```python
from build123d import *

# Parameters (mm, degrees)
F0_W     = 5
F0_H     = 5
F1_DEPTH = 3
F5_DEPTH = 5
F7_DEPTH = 7
F8_R     = 3.25
F9_DEPTH = 2


with BuildPart() as f1:
    # F0 (on Top) → F1 (new body)
    with BuildSketch(Plane.XY):
        with BuildLine():
            Line((2.5, 2.5), (5.4543560573, 2.5))
            ThreePointArc((5.4543560573, 2.5), (4.2426406871, 4.2426406871), (2.5, 5.4543560573))
            Line((2.5, 5.4543560573), (2.5, 2.5))
        make_face()
        with BuildLine():
            Line((2.5, -7.5), (2.5, -5.4543560573))
            ThreePointArc((2.5, -5.4543560573), (0, -6), (-2.5, -5.4543560573))
            Line((-2.5, -5.4543560573), (-2.5, -7.5))
            Line((-2.5, -7.5), (2.5, -7.5))
        make_face()
        with BuildLine():
            ThreePointArc((-5.4543560573, -2.5), (-4.2426406871, -4.2426406871), (-2.5, -5.4543560573))
            Line((-2.5, -5.4543560573), (-2.5, -2.5))
            Line((-2.5, -2.5), (-5.4543560573, -2.5))
        make_face()
        with BuildLine():
            ThreePointArc((-5.4543560573, -2.5), (-6, 0), (-5.4543560573, 2.5))
            Line((-5.4543560573, 2.5), (-7.5, 2.5))
            Line((-7.5, 2.5), (-7.5, -2.5))
            Line((-7.5, -2.5), (-5.4543560573, -2.5))
        make_face()
        with BuildLine():
            ThreePointArc((2.5, -5.4543560573), (4.2426406871, -4.2426406871), (5.4543560573, -2.5))
            Line((5.4543560573, -2.5), (2.5, -2.5))
            Line((2.5, -2.5), (2.5, -5.4543560573))
        make_face()
        with BuildLine():
            Line((-2.5, 2.5), (-2.5, 5.4543560573))
            ThreePointArc((-2.5, 5.4543560573), (-4.2426406871, 4.2426406871), (-5.4543560573, 2.5))
            Line((-5.4543560573, 2.5), (-2.5, 2.5))
        make_face()
        with BuildLine():
            ThreePointArc((5.4543560573, -2.5), (5.8620020617, -1.2794263668), (6, 0))
            ThreePointArc((6, 0), (5.8620020617, 1.2794263668), (5.4543560573, 2.5))
            Line((5.4543560573, 2.5), (2.5, 2.5))
            Line((2.5, 2.5), (2.5, -2.5))
            Line((2.5, -2.5), (5.4543560573, -2.5))
        make_face()
        Rectangle(F0_W, F0_H)
        with BuildLine():
            Line((-2.5, -2.5), (-2.5, 2.5))
            Line((-2.5, 2.5), (-5.4543560573, 2.5))
            ThreePointArc((-5.4543560573, 2.5), (-6, 0), (-5.4543560573, -2.5))
            Line((-5.4543560573, -2.5), (-2.5, -2.5))
        make_face()
        with BuildLine():
            Line((2.5, 2.5), (2.5, 5.4543560573))
            ThreePointArc((2.5, 5.4543560573), (0, 6), (-2.5, 5.4543560573))
            Line((-2.5, 5.4543560573), (-2.5, 2.5))
            Line((-2.5, 2.5), (2.5, 2.5))
        make_face()
        with BuildLine():
            ThreePointArc((-2.5, 5.4543560573), (0, 6), (2.5, 5.4543560573))
            Line((2.5, 5.4543560573), (2.5, 7.5))
            Line((2.5, 7.5), (-2.5, 7.5))
            Line((-2.5, 7.5), (-2.5, 5.4543560573))
        make_face()
        with BuildLine():
            ThreePointArc((5.4543560573, 2.5), (5.8620020617, 1.2794263668), (6, 0))
            ThreePointArc((6, 0), (5.8620020617, -1.2794263668), (5.4543560573, -2.5))
            Line((5.4543560573, -2.5), (7.5, -2.5))
            Line((7.5, -2.5), (7.5, 2.5))
            Line((7.5, 2.5), (5.4543560573, 2.5))
        make_face()
        with BuildLine():
            ThreePointArc((-2.5, -5.4543560573), (0, -6), (2.5, -5.4543560573))
            Line((2.5, -5.4543560573), (2.5, -2.5))
            Line((2.5, -2.5), (-2.5, -2.5))
            Line((-2.5, -2.5), (-2.5, -5.4543560573))
        make_face()
    extrude(amount=F1_DEPTH)

    # F5 (add): a face of the model
    f5_faces = [f1.faces().sort_by_distance(p)[0] for p in [
        (0, 0, 0),
    ]]
    extrude(f5_faces, amount=F5_DEPTH)


with BuildPart() as f4:
    # F3 (on Right) → F4 (revolve)
    with BuildSketch(Plane.YZ):
        with BuildLine():
            Line((0, -12), (0, 0))
            ThreePointArc((0, 0), (-6, -6), (0, -12))
        make_face()
    revolve(axis=Axis((0, 0, -6), (0, 0, -1)))


with BuildPart() as f1_1:
    add(f1.part)

    # F6: cut F4
    add(f4.part, mode=Mode.SUBTRACT)

    # F2 (on face) → F7 (join)
    with BuildSketch(Plane.XY.offset(3)):
        with BuildLine():
            ThreePointArc((-2.5, 5.4543560573), (-4.2426406871, 4.2426406871), (-5.4543560573, 2.5))
            Line((-5.4543560573, 2.5), (-7.5, 2.5))
            Line((-7.5, 2.5), (-7.5, -2.5))
            Line((-7.5, -2.5), (-5.4543560573, -2.5))
            ThreePointArc((-5.4543560573, -2.5), (-4.2426406871, -4.2426406871), (-2.5, -5.4543560573))
            Line((-2.5, -5.4543560573), (-2.5, -7.5))
            Line((-2.5, -7.5), (2.5, -7.5))
            Line((2.5, -7.5), (2.5, -5.4543560573))
            ThreePointArc((2.5, -5.4543560573), (4.2426406871, -4.2426406871), (5.4543560573, -2.5))
            Line((5.4543560573, -2.5), (7.5, -2.5))
            Line((7.5, -2.5), (7.5, 2.5))
            Line((7.5, 2.5), (5.4543560573, 2.5))
            ThreePointArc((5.4543560573, 2.5), (4.2426406871, 4.2426406871), (2.5, 5.4543560573))
            Line((2.5, 5.4543560573), (2.5, 7.5))
            Line((2.5, 7.5), (-2.5, 7.5))
            Line((-2.5, 7.5), (-2.5, 5.4543560573))
        make_face()
    extrude(amount=F7_DEPTH)

    # F8 (on face) → F9 (cut)
    with BuildSketch(Plane.XY.offset(10)):
        Circle(F8_R)
    extrude(amount=-F9_DEPTH, mode=Mode.SUBTRACT)


solid = f1_1.part
```
Geometry check sheet. Reference: the model listing, model coordinates, mm. A direction names the side the tool comes from. Round coordinates to 2 decimals unless told otherwise and drop trailing zeros. Loops run counter-clockwise (first coordinate to the right, second up) from the corner with the lowest first, then second, coordinate; pieces in that order, holes last. Notation, with made-up numbers: (-35.5, 25) - (-28.5, 25) arc R17 cw to (-28.5, 39) - close; hole circle Ø5 at (38, 14). An arc over 180 degrees is marked (long way). Write each question's results on one line, items separated by ' | '. Start each with the question number.
Q1. Cross-section at A-A on x = 0. Enter the section's corners in (y, z), and give its area (3 significant figures).
Q2. Access from +Z, -Z, +X, -X, +Y, -Y to the whole of each face (thin tool, end or side, straight path). Record for faces 1 (the flat face through (2.5, 6, 2)), 2 (the flat face through (0, 0, 8)), 3 (the flat face through (6, -2.5, 2)).
Q3. Cross-section at B-B on z = 8.5. Enter the section's corners in (x, y), and give its area (3 significant figures).
Q4. Release check for a two-part mould opening along X. For faces 4 (the flat face through (7.5, 0, 2)), 5 (the flat face through (-2.5, -6, 2)), 6 (the cylindrical face through (-2.579, -1.978, 9.014)) record: +X half, -X half, draft (parallel to the pull), parting line (faces both ways), or undercut.
Q5. Gauge pin test, flat ends, axial feed: P1, Ø1.5, axis at x = 1, y = -0.5, coming from the +Z side; P2, Ø1, axis at y = 6, z = 0, coming from the -X side; P3, Ø2.5, axis at y = -6, z = 3, coming from the -X side; P4, Ø1, axis at x = -4, y = 6, coming from the +Z side. Record the tip position at first contact, or that the pin passes through.
Q6. Thickness scan on line 1 (Y direction, x = 0, z = 9); line 2 (Y direction, x = -5.75, z = -0.5); line 3 (X direction, y = 4, z = -2.5). Record the ranges inside material, lowest first. Write a range as [from, to].
Q7. Cross-section at D-D on z = 3.5. Enter the section's corners in (x, y), and give its area (3 significant figures).
Answers below:
1) outline: (-7.5, -5) - (-5.92, -5) arc R6 cw to (5.92, -5) - (7.5, -5) - (7.5, 10) - (3.25, 10) - (3.25, 8) - (-3.25, 8) - (-3.25, 10) - (-7.5, 10) - close | area: 167 mm²
2) face 1: +Z, -Z, +X, +Y | face 2: +Z | face 3: +Z, -Z, +X, -Y
3) outline: (-7.5, -2.5) - (-5.45, -2.5) arc R6 ccw to (-2.5, -5.45) - (-2.5, -7.5) - (2.5, -7.5) - (2.5, -5.45) arc R6 ccw to (5.45, -2.5) - (7.5, -2.5) - (7.5, 2.5) - (5.45, 2.5) arc R6 ccw to (2.5, 5.45) - (2.5, 7.5) - (-2.5, 7.5) - (-2.5, 5.45) arc R6 ccw to (-5.45, 2.5) - (-7.5, 2.5) - close; hole circle Ø6.5 at (0, 0) | area: 113 mm²
4) face 4: +X half | face 5: -X half | face 6: undercut
5) P1: stops at z = 8 | P2: stops at x = -2.5 | P3: stops at x = -3.67 | P4: passes through
6) line 1: y = [-7.5, -3.25], [3.25, 7.5] | line 2: y = [-2.5, 2.5] | line 3: x = [-4.47, -2.78], [2.78, 4.47]
7) outline: (-7.5, -2.5) - (-5.45, -2.5) arc R6 ccw to (-2.5, -5.45) - (-2.5, -7.5) - (2.5, -7.5) - (2.5, -5.45) arc R6 ccw to (5.45, -2.5) - (7.5, -2.5) - (7.5, 2.5) - (5.45, 2.5) arc R6 ccw to (2.5, 5.45) - (2.5, 7.5) - (-2.5, 7.5) - (-2.5, 5.45) arc R6 ccw to (-5.45, 2.5) - (-7.5, 2.5) - close | area: 147 mm²
